Check sheet for the modelled part. Datum: model origin and axes. Units: mm. Round coordinates to 2 decimals unless told otherwise and drop trailing zeros. Order: outer loops, then holes, each group sorted by start corner. A loop starts at its lowest first (then second) coordinate and runs counter-clockwise, first axis right, second up. Notation, with made-up numbers: (25.5, -7.5) -> (57.5, -7.5) arc R13 cw to (57.5, 5.5) -> close; hole circle Ø1 at (40, 75.25). An arc over 180 degrees is marked (long way). Answer in a Markdown table with one row per item. Add a question column.
1. Depth check by flat-ended pin: P1, Ø1, axis at x = -15.5, y = -71.5, coming from the +Z side; P2, Ø5, axis at x = 310, y = -26, coming from the -Z side; P3, Ø8, axis at x = 35.5, y = -103.5, coming from the -Z side. Enter the tip coordinate at first touch or a pass-through.
2. Sectioned sample at A-A, the plane z = 0. Record the boundary of the cut face in (x, y).
3. Sectioned sample at B-B, the plane x = 0. Record the boundary of the cut face in (y, z).
4. Material ranges on L1, parallel to X at y = -15, z = 0; L2, parallel to X at y = -9.5, z = 232; L3, parallel to Z at x = 0, y = -30, recorded low to high. Write a range as from..to.
5. Sectioned sample at C-C, the plane y = -22. Record the boundary of the cut face in (x, z), then the cut area to 3 significant figures.
```python
from build123d import *

# Parameters (mm, degrees)
F3_W     = 673.8248765469
F3_H     = 114.0088248253
F4_DEPTH = 253


with BuildPart() as f2:
    # F1 (on Right) → F2 (revolve)
    with BuildSketch(Plane.YZ):
        Polygon((0, 474.8347821527), (0, 499.8347821527), (-34.02, 499.8347821527), (-63.8654725708, 474.8347821527), align=None)
    revolve(axis=Axis((0, 1.7310532815, 0), (0, -1, 0)))

    # F3 (on Front) → F4 (cut)
    with BuildSketch(Plane.XZ):
        with Locations((0.930711627, -452.0044124126)):
            Rectangle(F3_W, F3_H)
    extrude(amount=F4_DEPTH, mode=Mode.SUBTRACT)

    # F8: sweep along a path in F6
    with BuildLine(Plane.XY.offset(-395)) as f8_path:
        ThreePointArc((263.5205311585, 0), (0, -65.2754158494), (-263.5205311585, 0))
    # F7 (on Right) → F8 (sweep)
    with BuildSketch(Plane.YZ):
        Polygon((-65.2754158494, -395), (-65.2754158494, -370), (-127.0850614031, -370), (-99.2954158494, -395), align=None)
    sweep(path=f8_path.line)


solid = f2.part
```
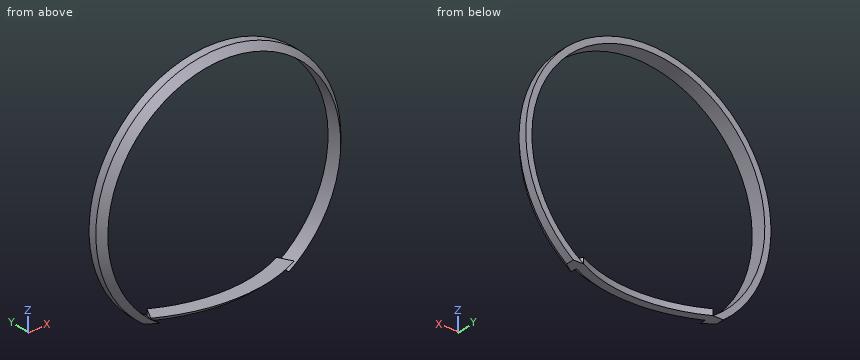
Answer key:
| question | item | result |
|---|---|---|
| 1 | P1 | stops at z = -370 |
| 1 | P2 | stops at z = -394.05 |
| 1 | P3 | stops at z = -393.88 |
| 2 | outline | (-499.83, -34.02) -> (-474.83, -63.87) -> (-474.83, 0) -> (-499.83, 0) -> close; (474.83, -63.87) -> (499.83, -34.02) -> (499.83, 0) -> (474.83, 0) -> close |
| 3 | outline | (-127.09, -370) -> (-99.3, -395) -> (-65.28, -395) -> (-65.28, -370) -> close; (-63.87, 474.83) -> (0, 474.83) -> (0, 499.83) -> (-34.02, 499.83) -> close |
| 4 | L1 | x = -499.83..-474.83, 474.83..499.83 |
| 4 | L2 | x = -442.73..-414.3, 414.3..442.73 |
| 4 | L3 | z = 474.83..499.83 |
| 5 | outline | (-306.28, -395) -> (-216.77, -395) -> (-216.77, -370) -> (-275.13, -370) -> (-275.13, -387) arc R474.83 cw (long way) to (275.13, -387) -> (275.13, -370) -> (216.77, -370) -> (216.77, -395) -> (306.28, -395) arc R499.83 ccw (long way) to start |
| 5 | area | 64,100 mm² |
